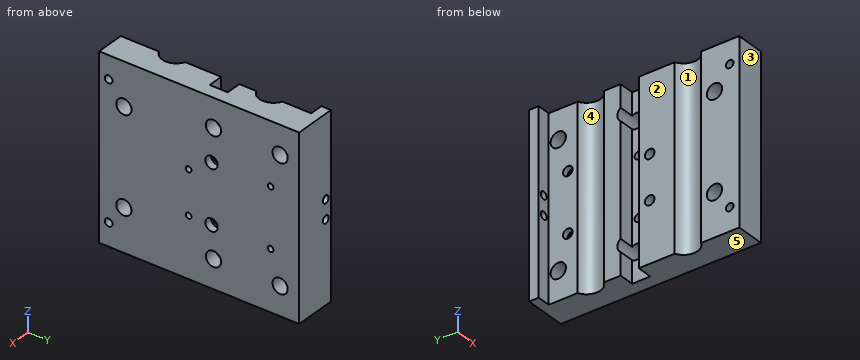
```python
from build123d import *

# Parameters (mm, degrees)
BOSS_EXTRUDE1_DEPTH                = 95
SKETCH2_R                          = 2
CUT_EXTRUDE1_3DPRINTER4_DEPTH      = 139.744369255
ESQUISSE1_R                        = 1.5
ENL_V_MAT_EXTRU_1_3D_PRINTER_DEPTH = 140.67462189
ENL_V_MAT_EXTRU_2_DEPTH            = 139.744369255
ENL_V_MAT_EXTRU_2_DEPTH_BACK       = 3
ESQUISSE2_R                        = 2.5
ESQUISSE3_R                        = 3.25
ENL_V_MAT_EXTRU_3_DEPTH            = 4
ESQUISSE4_R                        = 2
ENL_V_MAT_EXTRU_4_DEPTH            = 140.67462189
ESQUISSE8_R                        = 7.5
ENL_V_MAT_EXTRU_9_DEPTH            = 139.744369255
ESQUISSE9_R                        = 4
ENL_V_MAT_EXTRU_10CNC_TROUS_DEPTH  = 140.67462189
ESQUISSE10_R                       = 2
ENL_V_MAT_EXTRU_10_DEPTH           = 139.744369255
ESQUISSE11_R                       = 2.5
ENL_V_MAT_EXTRU_11_DEPTH           = 5


with BuildPart() as part:
    # Sketch1 → Boss-Extrude1 (new body)
    with BuildSketch(Plane.XY):
        Polygon((0, 0), (0, -37.75), (8, -37.75), (8, -47.25), (0, -47.25), (0, -100), (15, -100), (15, 5), (-7, 5), (-7, 0), align=None)
    extrude(amount=BOSS_EXTRUDE1_DEPTH)

    # Sketch2 → Cut-Extrude1 3dprinter4 (cut, through all)
    with BuildSketch(Plane.ZY):
        with Locations(Location((62.5, -41, 0), (0, 0, 270))):
            Circle(SKETCH2_R)
        with Locations(Location((31.5, -41, 0), (0, 0, 270))):
            Circle(SKETCH2_R)
    extrude(amount=-CUT_EXTRUDE1_3DPRINTER4_DEPTH, mode=Mode.SUBTRACT)

    # Esquisse1 → Enlèv. mat.-Extru.1 3d printer (cut, through all)
    with BuildSketch(Plane(origin=(15, 0, 0), x_dir=(0, 0, -1), z_dir=(1, 0, 0))):
        with Locations(Location((-62.5, -10, 0), (0, 0, 90))):
            Circle(ESQUISSE1_R)
        with Locations(Location((-31.5, -10, 0), (0, 0, 90))):
            Circle(ESQUISSE1_R)
        with Locations(Location((-54.5, -53, 0), (0, 0, 90))):
            Circle(ESQUISSE1_R)
        with Locations(Location((-31.5, -53, 0), (0, 0, 90))):
            Circle(ESQUISSE1_R)
    extrude(amount=-ENL_V_MAT_EXTRU_1_3D_PRINTER_DEPTH, mode=Mode.SUBTRACT)

    # Esquisse2 → Enlèv. mat.-Extru.2 (cut, two sides: drawn at the far end of the back side and taken through both)
    with BuildSketch(Plane.ZY.offset(-ENL_V_MAT_EXTRU_2_DEPTH_BACK)):
        with Locations(Location((62.5, -10, 0), (0, 0, 90))):
            Circle(ESQUISSE2_R)
        with Locations(Location((31.5, -10, 0), (0, 0, 90))):
            Circle(ESQUISSE2_R)
    extrude(amount=ENL_V_MAT_EXTRU_2_DEPTH + ENL_V_MAT_EXTRU_2_DEPTH_BACK, mode=Mode.SUBTRACT)

    # Esquisse3 → Enlèv. mat.-Extru.3 (cut)
    with BuildSketch(Plane(origin=(15, 0, 0), x_dir=(0, 0, -1), z_dir=(1, 0, 0))):
        with Locations(Location((-31.5, -41, 0), (0, 0, 90))):
            Circle(ESQUISSE3_R)
        with Locations(Location((-62.5, -41, 0), (0, 0, 90))):
            Circle(ESQUISSE3_R)
    extrude(amount=-ENL_V_MAT_EXTRU_3_DEPTH, mode=Mode.SUBTRACT)

    # Esquisse4 → Enlèv. mat.-Extru.4 (cut, through all)
    with BuildSketch(Plane(origin=(15, 0, 0), x_dir=(0, 0, -1), z_dir=(1, 0, 0))):
        with Locations(Location((-83, -95, 0), (0, 0, 90))):
            Circle(ESQUISSE4_R)
        with Locations(Location((-12, -95, 0), (0, 0, 90))):
            Circle(ESQUISSE4_R)
    extrude(amount=-ENL_V_MAT_EXTRU_4_DEPTH, mode=Mode.SUBTRACT)

    # Esquisse8 → Enlèv. mat.-Extru.9 (cut, through all)
    with BuildSketch(Plane(origin=(0, 0, 0), x_dir=(-1, 0, 0), z_dir=(0, 0, -1))):
        with Locations((3, -22)):
            Circle(ESQUISSE8_R)
        with Locations((3, -73)):
            Circle(ESQUISSE8_R)
    extrude(amount=-ENL_V_MAT_EXTRU_9_DEPTH, mode=Mode.SUBTRACT)

    # Esquisse9 → Enlèv. mat.-Extru.10cnc trous (cut, through all)
    with BuildSketch(Plane(origin=(15, 0, 0), x_dir=(0, 0, -1), z_dir=(1, 0, 0))):
        with Locations(Location((-15, -5, 0), (0, 0, 90))):
            Circle(ESQUISSE9_R)
        with Locations(Location((-80, -5, 0), (0, 0, 90))):
            Circle(ESQUISSE9_R)
        with Locations(Location((-80, -40, 0), (0, 0, 90))):
            Circle(ESQUISSE9_R)
        with Locations(Location((-15, -40, 0), (0, 0, 90))):
            Circle(ESQUISSE9_R)
        with Locations(Location((-22.5, -87, 0), (0, 0, 90))):
            Circle(ESQUISSE9_R)
        with Locations(Location((-72.5, -87, 0), (0, 0, 90))):
            Circle(ESQUISSE9_R)
    extrude(amount=-ENL_V_MAT_EXTRU_10CNC_TROUS_DEPTH, mode=Mode.SUBTRACT)

    # Esquisse10 → Enlèv. mat.-Extru.10 (cut, through all)
    with BuildSketch(Plane.XZ):
        with Locations(Location((-3.5, 52.5, 0), (0, 0, 270))):
            Circle(ESQUISSE10_R)
        with Locations(Location((-3.5, 42.5, 0), (0, 0, 270))):
            Circle(ESQUISSE10_R)
    extrude(amount=-ENL_V_MAT_EXTRU_10_DEPTH, mode=Mode.SUBTRACT)

    # Esquisse11 → Enlèv. mat.-Extru.11 (cut)
    with BuildSketch(Plane.ZY):
        with Locations(Location((54.5, -53, 0), (0, 0, 270))):
            Circle(ESQUISSE11_R)
        with Locations(Location((31.5, -53, 0), (0, 0, 270))):
            Circle(ESQUISSE11_R)
    extrude(amount=-ENL_V_MAT_EXTRU_11_DEPTH, mode=Mode.SUBTRACT)


solid = part.part
```
The model under review builds one solid part; all positions refer to its coordinate system, in mm. Face numbers are marked on the shaded views. A direction names the side the tool comes from. Round coordinates to 2 decimals unless told otherwise and drop trailing zeros. Write each loop counter-clockwise with the first axis right and the second up, starting at its lowest first coordinate (ties: lowest second). Pieces come first, ordered by that corner, then holes. Notation, with made-up numbers: (48, 85.25) - (105, 85.25) arc R24 cw to (105, 105.25) - close; hole circle Ø3 at (45.5, -39). An arc over 180 degrees is marked (long way). One line per question, with ' | ' between items.
Item 1: Add section B-B, the plane x = 1.75. State how many separate pieces and enclosed holes the cut face has, then the cut area to 3 significant figures.
Resolved:
separate pieces: 4 | enclosed holes: 10 | area: 6,550 mm2
Item 2: To check wall thickness, follow probe 1 along Z at (x, y) = (9.25, -5); probe 2 along Z at (x, y) = (12, -95); probe 3 along Y at (x, z) = (7.5, 32). State the ranges of each line that lie inside material, in increasing order.
Resolved:
probe 1: z = 0 to 11, 19 to 76, 84 to 95 | probe 2: z = 0 to 10, 14 to 81, 85 to 95 | probe 3: y = -100 to -54.41, -51.59 to -47.25, -37.75 to -11.41, -8.59 to 5
Item 3: For P1, Ø6.5, axis at y = -53, z = 54.5, coming from the -X side; P2, Ø2.5, axis at y = -53.5, z = 32, coming from the -X side; P3, Ø2, axis at y = -40.5, z = 64, coming from the +X side, all flat-tipped, find the tip position at first contact; note any pin that passes through.
Resolved:
P1: stops at x = 0 | P2: stops at x = 5 | P3: stops at x = 11
Item 4: For the marked faces 1 and 2, list the 3-axis set-ups (+Z, -Z, +X, -X, +Y, -Y) from which the entire face can be reached by the end or side of a thin tool; tool diameter is ignored.
Resolved:
face 1: +Z, -Z, -X | face 2: +Z, -Z, -X, -Y
Item 5: Add section A-A, the plane z = 42.5. Give the boundary of the cut face in (x, y).
Resolved:
outline: (-7, 0) - (-5.5, 0) - (-5.5, 5) - (-7, 5) - close; (-1.5, 0) - (0, 0) - (0, -15.13) arc R7.5 cw to (0, -28.87) - (0, -37.75) - (8, -37.75) - (8, -47.25) - (0, -47.25) - (0, -66.13) arc R7.5 cw to (0, -79.87) - (0, -100) - (15, -100) - (15, 5) - (-1.5, 5) - close
Item 6: The part is to be moulded in two halves that separate along Y. For the marked faces 3, 4 and 5, say which applies: pulls with the +Y half, pulls with the -Y half, needs draft (parallel to the pull), parting line crosses it, or undercut.
Resolved:
face 3: pulls with the -Y half | face 4: undercut | face 5: needs draft
Item 7: Add section C-C, the plane y = -53. Give the boundary of the cut face in (x, z).
Resolved:
outline: (0, 0) - (15, 0) - (15, 30) - (5, 30) - (5, 29) - (0, 29) - close; (0, 34) - (5, 34) - (5, 33) - (15, 33) - (15, 53) - (5, 53) - (5, 52) - (0, 52) - close; (0, 57) - (5, 57) - (5, 56) - (15, 56) - (15, 95) - (0, 95) - close
